Autodesk Inventor part; units mm, degrees
ref_plane "YZ Plane" through (0, 0, 0) normal (1, 0, 0) x (0, 1, 0)
ref_plane "XZ Plane" through (0, 0, 0) normal (0, 1, 0) x (-1, 0, 0)
ref_plane "XY Plane" through (0, 0, 0) normal (0, 0, 1) x (1, 0, 0)
sketch "Sketch1" plane through (0, 0, 0) normal (0, 0, 1) x (1, 0, 0)
  line L0 (-50, 55) -> (50, 55)
  line L1 (50, 55) -> (50, -55)
  line L2 (50, -55) -> (-50, -55)
  line L3 (-50, -55) -> (-50, 55)
  line L4 (-50, 55) -> (50, -55) construction
  line L5 (50, 55) -> (-50, -55) construction
  point P0 (0, 0)
  dimension "d0" = 100
  dimension "d1" = 110
extrude "Extrusion1" add sketch "Sketch1" along normal blind 1.8
sketch "Sketch2" plane through (0, 0, 1.8) normal (0, 0, 1) x (1, 0, 0)
  line L0 (-26.5, -21.4) -> (-7.5, -21.4)
  line L1 (-7.5, -21.4) -> (-7.5, -40.4)
  line L2 (-7.5, -40.4) -> (-26.5, -40.4)
  line L3 (-26.5, -40.4) -> (-26.5, -21.4)
  line L4 (-26.5, -21.4) -> (-7.5, -40.4) construction
  line L5 (-7.5, -21.4) -> (-26.5, -40.4) construction
  line L6 (-50, -55) -> (50, -55)
  line L7 (-50, 55) -> (-50, -55)
  point P0 (0, 0)
  point P1 (-17, -30.9)
  dimension "d4" = 19
  dimension "d5" = 19
  dimension "d8" = 33.6
  dimension "d9" = 42.5
extrude "Extrusion2" add sketch "Sketch2" along normal blind 1
pattern_linear "Rectangular Pattern1" count 2 spacing 31 along (1, 0, 0) count 2 spacing 27 along (0, 1, 0) of "Extrusion2"
sketch "Sketch3" plane through (0, 0, 1.8) normal (0, 0, 1) x (1, 0, 0)
  line L0 (-46.7, -46.1) -> (-26.7, -46.1) construction
  line L1 (-46.7, -47.2) -> (-26.7, -47.2)
  line L2 (-26.7, -45) -> (-46.7, -45)
  arc A0 (-46.7, -45) -> (-46.7, -47.2) centre (-46.7, -46.1) ccw
  arc A1 (-26.7, -47.2) -> (-26.7, -45) centre (-26.7, -46.1) ccw
  line L3 (-50, 55) -> (-50, -55)
  line L4 (-50, -55) -> (50, -55)
  point P0 (0, 0)
  point P1 (-36.7, -46.1)
  dimension "d16" = 20
  dimension "d17" = 2.2
  dimension "d18" = 2.2
  dimension "d19" = 7.8
extrude "Extrusion3" cut sketch "Sketch3" against normal through all
pattern_linear "Rectangular Pattern2" count 4 spacing 24.6 along (1, 0, 0) count 2 spacing 92 along (0, 1, 0) of "Extrusion3"
sketch "Sketch4" plane through (0, 0, 1.8) normal (0, 0, 1) x (1, 0, 0)
  line L0 (50, -55) -> (50, 55)
  line L1 (50, 42.3) -> (-50.0933, 42.3) construction
  line L2 (47.1, 44.8) -> (27.1, 44.8)
  line L3 (50, -5.2) -> (-50.0933, -5.2) construction
  line L4 (35, 55) -> (35, -55) construction
  line L5 (36, 55) -> (36, -55) construction
  line L6 (-47, 55) -> (-47, -55) construction
  line L7 (-50, -55) -> (50, -55) construction
  line L8 (-50, 55) -> (-50, -55) construction
  line L9 (-50, 23) -> (-32.5921, 23) construction
  line L10 (50, 55) -> (-50, 55) construction
  line L11 (60.1599, 62.0026) -> (59.0568, -63.0375) construction
  line L12 (59.0568, -63.0375) -> (-57.4953, -62.0093) construction
  line L13 (-57.4953, -62.0093) -> (-56.3922, 63.0308) construction
  line L14 (-56.3922, 63.0308) -> (60.1599, 62.0026) construction
  point P0 (0, 0)
  dimension "d28" = 2.5
  dimension "d29" = 50
  dimension "d30" = 15
  dimension "d31" = 14
  dimension "d44" = 3
  dimension "d45" = 32
sketch "Sketch5" plane through (0, 0, 1.8) normal (0, 0, 1) x (1, 0, 0)
  line L0 (-50, 55) -> (-50, -55)
  line L1 (50, -55) -> (50, 55)
  line L2 (50, 55) -> (-50, 55)
  line L3 (-50, -55) -> (50, -55)
  point P0 (0, 0)
  point P1 (-40, 51)
  point P2 (41, 51)
  point P3 (-40, -51)
  point P4 (40, -51)
  dimension "d32" = 10
  dimension "d33" = 9
  dimension "d34" = 4
  dimension "d36" = 4
  dimension "d88" = 10
hole "Hole1" at (-40, 51, 1.8) at (-40, -51, 1.8) at (40, -51, 1.8) at (41, 51, 1.8) direction (0, 0, -1) diameter 3 end through all
sketch "Sketch7" plane through (0, 0, 1.8) normal (0, 0, 1) x (1, 0, 0)
  point P0 (0, 0)
properties part number "PCB"
Could you check a few things on this model? Use its own coordinates, in mm. Give positions to 0.01 mm unless a question says otherwise; leave off trailing zeros. Order: outer loops, then holes, each group sorted by start corner. A loop starts at its lowest first (then second) coordinate and runs counter-clockwise, first axis right, second up. Notation, with made-up numbers: (-26, 66) - (-2, 66) arc R20 cw to (-2, 77) - close; hole circle Ø9 at (47, 88.25). An arc over 180 degrees is marked (long way). One line per question, with ' | ' between items. Start each with the question number.
Item 1: I want a section at D-D on z = 0.7. Give the number of separate pieces and of enclosed holes in the cut face, then the cut area to 3 significant figures.
Item 2: I want a section at A-A on x = -20.5. Write out the boundary of the cut face in (y, z), then the cut area to 3 significant figures.
Item 3: I want a section at B-B on y = -51. Write out the boundary of the cut face in (x, z), then the cut area to 3 significant figures.
Item 4: I'm going to push flat-ended pins straight in: pin 1 Ø4 at (x, y) = (40, -51) entering from +Z; pin 2 Ø0.5 at (x, z) = (-16.5, 2.5) entering from -Y; pin 3 Ø0.5 at (x, z) = (-15, 2.5) entering from +Y; pin 4 Ø1.8 at (x, y) = (41, 51) entering from -Z. Where does each tip first touch, or does it pass through?
Item 5: I want a section at C-C on x = -40. Write out the boundary of the cut face in (y, z), then the cut area to 3 significant figures.
Item 6: I need wall thicknesses on probe 1 along Y at (x, z) = (-31, 0.5); probe 2 along X at (y, z) = (-51, 0.7); probe 3 along Y at (x, z) = (-40, 1.35). Which ranges of each line are inside material? Lowest first, please. Write a range as [from, to].
Item 7: Thinking about a two-plate mould opening in Y: for faces 1 (the flat face through (-1, 1, 0)), 2 (the cylindrical face through (40.9, -49.8, 0.9)), which applies, pulls with the +Y half, pulls with the -Y half, needs draft (parallel to the pull), parting line crosses it, or undercut?
Verdict:
1) separate pieces: 1 | enclosed holes: 12 | area: 10,600 mm^2
2) outline: (-55, 0) - (-47.2, 0) - (-47.2, 1.8) - (-55, 1.8) - close; (-45, 0) - (44.8, 0) - (44.8, 1.8) - (5.6, 1.8) - (5.6, 2.8) - (-13.4, 2.8) - (-13.4, 1.8) - (-21.4, 1.8) - (-21.4, 2.8) - (-40.4, 2.8) - (-40.4, 1.8) - (-45, 1.8) - close; (47, 0) - (55, 0) - (55, 1.8) - (47, 1.8) - close | area: 228 mm^2
3) outline: (-50, 0) - (-41.5, 0) - (-41.5, 1.8) - (-50, 1.8) - close; (-38.5, 0) - (38.5, 0) - (38.5, 1.8) - (-38.5, 1.8) - close; (41.5, 0) - (50, 0) - (50, 1.8) - (41.5, 1.8) - close | area: 169 mm^2
4) pin 1: z = 1.8 | pin 2: y = -40.4 | pin 3: y = 5.6 | pin 4: through
5) outline: (-55, 0) - (-52.5, 0) - (-52.5, 1.8) - (-55, 1.8) - close; (-49.5, 0) - (-47.2, 0) - (-47.2, 1.8) - (-49.5, 1.8) - close; (-45, 0) - (44.8, 0) - (44.8, 1.8) - (-45, 1.8) - close; (47, 0) - (49.5, 0) - (49.5, 1.8) - (47, 1.8) - close; (52.5, 0) - (55, 0) - (55, 1.8) - (52.5, 1.8) - close | area: 179 mm^2
6) probe 1: [-55, -47.2], [-45, 44.8], [47, 55] | probe 2: [-50, -41.5], [-38.5, 38.5], [41.5, 50] | probe 3: [-55, -52.5], [-49.5, -47.2], [-45, 44.8], [47, 49.5], [52.5, 55]
7) face 1: needs draft | face 2: undercut
